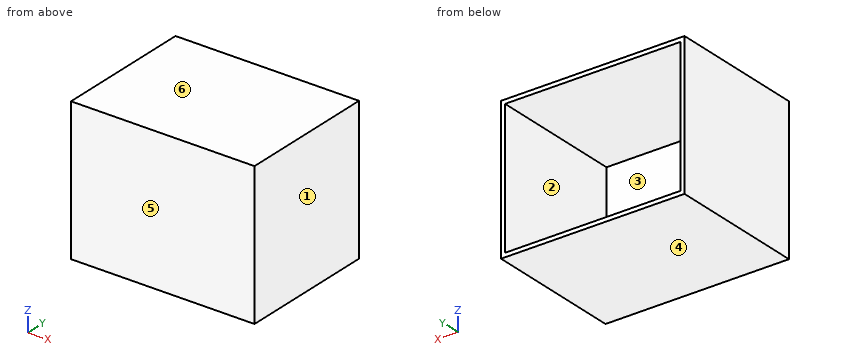
Autodesk Inventor part; units mm, degrees
ref_plane "YZ Plane" through (0, 0, 0) normal (1, 0, 0) x (0, 1, 0)
ref_plane "XZ Plane" through (0, 0, 0) normal (0, 1, 0) x (-1, 0, 0)
ref_plane "XY Plane" through (0, 0, 0) normal (0, 0, 1) x (1, 0, 0)
sketch "Sketch1" plane through (0, 0, 0) normal (0, 1, 0) x (-1, 0, 0)
  line L0 (0, 0) -> (-136, 0)
  line L1 (-136, 0) -> (-136, 106)
  line L2 (-136, 106) -> (0, 106)
  line L3 (0, 106) -> (0, 0)
  dimension "d0" = 106
  dimension "d1" = 136
extrude "Extrusion1" add sketch "Sketch1" along normal blind 3
sketch "Sketch2" plane through (0, 3, 0) normal (0, 1, 0) x (1, 0, 0)
  line L0 (3, -3) -> (133, -3)
  line L1 (133, -3) -> (133, -103)
  line L2 (133, -103) -> (3, -103)
  line L3 (3, -103) -> (3, -3)
  line L4 (0, 0) -> (0, -106)
  line L5 (136, 0) -> (0, 0)
  line L6 (0, -106) -> (136, -106)
  line L7 (0, 0) -> (136, 0)
  line L8 (136, 0) -> (136, -106)
  line L9 (136, -106) -> (0, -106)
  line L10 (0, -106) -> (0, 0)
  dimension "d4" = 130
  dimension "d5" = 100
  dimension "d6" = 3
  dimension "d7" = 3
extrude "Extrusion2" add sketch "Sketch2" along normal blind 100
properties part number "case"
Design review of the part built by this model. Coordinates are the model's own, in mm. Face numbers are marked on the shaded views. A direction names the side the tool comes from. Give positions to 0.01 mm unless a question says otherwise; leave off trailing zeros. Order: outer loops, then holes, each group sorted by start corner. A loop starts at its lowest first (then second) coordinate and runs counter-clockwise, first axis right, second up. Notation, with made-up numbers: (47.5, 33) -> (75.5, 33) arc R18 ccw to (75.5, 59) -> close; hole circle Ø8 at (-20.75, -31). An arc over 180 degrees is marked (long way). Write each question's results on one line, items separated by ' | '. Start each with the question number.
Q1. Wall thickness on L1, parallel to X at y = 40, z = 16.5; L2, parallel to Z at x = 103, y = 53; L3, parallel to Y at x = 80.5, z = 54: over which ranges is each line inside the solid? List them lowest first. Write a range as from..to.
Q2. For pin 1 (2 mm diameter, centred on x = 105.5, z = 83.5, fed in from +Y), flat-tipped, find the tip position at first contact; note if it passes through.
Q3. Add section C-C on x = 39. Give the boundary of the cut face in (y, z).
Q4. Mouldability with a two-part tool opening along Z and no side actions: class the marked faces 3, 4, 5 and 6 as +Z half, -Z half, draft (parallel to the pull), parting line (faces both ways), or undercut.
Q5. Machinability: for the marked faces 1 and 2, which of the approach directions +Z, -Z, +X, -X, +Y, -Y give a long, thin tool a straight path to every point of the face, cutting with its end or side? Answer none if there is none.
Q6. Add section B-B on z = 77. Give the boundary of the cut face in (x, y), and give its area (3 significant figures).
Q7. Add section A-A on y = 55.5. Give the boundary of the cut face in (x, z), and give its area (3 significant figures).
Found:
1) L1: x = 0..3, 133..136 | L2: z = 0..3, 103..106 | L3: y = 0..3
2) pin 1: stops at y = 3
3) outline: (0, 0) -> (103, 0) -> (103, 3) -> (3, 3) -> (3, 103) -> (103, 103) -> (103, 106) -> (0, 106) -> close
4) face 3: undercut | face 4: -Z half | face 5: draft | face 6: +Z half
5) face 1: +Z, -Z, +X, +Y, -Y | face 2: +Y
6) outline: (0, 0) -> (136, 0) -> (136, 103) -> (133, 103) -> (133, 3) -> (3, 3) -> (3, 103) -> (0, 103) -> close | area: 1,010 mm2
7) outline: (0, 0) -> (136, 0) -> (136, 106) -> (0, 106) -> close; hole (3, 3) -> (133, 3) -> (133, 103) -> (3, 103) -> close | area: 1,420 mm2
